from build123d import *

# Parameters (mm, degrees)
ESQUISSE1_W                  = 18.3
ESQUISSE1_H                  = 17.8
BOSS_EXTRU_1_DEPTH           = 34.4
ENL_V_MAT_EXTRU_1_DEPTH      = 37.69185877
ENL_V_MAT_EXTRU_1_DEPTH_BACK = 37.69185877
ENL_V_MAT_EXTRU_2_DEPTH      = 37.69185877
ENL_V_MAT_EXTRU_2_DEPTH_BACK = 37.69185877
ESQUISSE4_R                  = 4.25
BOSS_EXTRU_2_DEPTH           = 2.2
ESQUISSE5_R                  = 2.45
BOSS_EXTRU_3_DEPTH           = 2.1
BOSS_EXTRU_4_DEPTH           = 1.3
ESQUISSE7_R                  = 1.85
BOSS_EXTRU_5_DEPTH           = 10.3
ESQUISSE8_R                  = 6.5
ESQUISSE8_R_2                = 6.1
ENL_V_MAT_EXTRU_3_DEPTH      = 0.1


with BuildPart() as part:
    # Esquisse1 → Boss.-Extru.1 (new body)
    with BuildSketch(Plane(origin=(0, 0, 0), x_dir=(1, 0, 0), z_dir=(0, 1, 0))):
        Rectangle(ESQUISSE1_W, ESQUISSE1_H)
    extrude(amount=-BOSS_EXTRU_1_DEPTH)

    # Esquisse2 → Enlèv. mat.-Extru.1 (cut, two sides: drawn at the far end of the back side and taken through both)
    with BuildSketch(Plane(origin=(0, 0, 0), x_dir=(0, 0, -1), z_dir=(1, 0, 0)).offset(-ENL_V_MAT_EXTRU_1_DEPTH_BACK)):
        Polygon((8.9, -17.6), (4.4, -22.1), (4.4, -34.4), (8.9, -34.4), align=None)
    extrude(amount=ENL_V_MAT_EXTRU_1_DEPTH + ENL_V_MAT_EXTRU_1_DEPTH_BACK, mode=Mode.SUBTRACT)

    # Esquisse3 → Enlèv. mat.-Extru.2 (cut, two sides: drawn at the far end of the back side and taken through both)
    with BuildSketch(Plane.XY.offset(-ENL_V_MAT_EXTRU_2_DEPTH_BACK)):
        with BuildLine():
            Line((3.9, -30.7), (3.9, -25.7))
            ThreePointArc((3.9, -25.7), (5.4, -24.2), (6.9, -25.7))
            Line((6.9, -25.7), (6.9, -30.7))
            ThreePointArc((6.9, -30.7), (5.4, -32.2), (3.9, -30.7))
        make_face()
        with BuildLine():
            Line((-3.9, -30.7), (-3.9, -25.7))
            ThreePointArc((-3.9, -25.7), (-5.4, -24.2), (-6.9, -25.7))
            Line((-6.9, -25.7), (-6.9, -30.7))
            ThreePointArc((-6.9, -30.7), (-5.4, -32.2), (-3.9, -30.7))
        make_face()
    extrude(amount=ENL_V_MAT_EXTRU_2_DEPTH + ENL_V_MAT_EXTRU_2_DEPTH_BACK, mode=Mode.SUBTRACT)

    # Esquisse4 → Boss.-Extru.2 (add)
    with BuildSketch(Plane(origin=(0, 0, -4.4), x_dir=(-1, 0, 0), z_dir=(0, 0, -1))):
        with Locations((0, -19.85)):
            Circle(ESQUISSE4_R)
    extrude(amount=BOSS_EXTRU_2_DEPTH)

    # Esquisse5 → Boss.-Extru.3 (add)
    with BuildSketch(Plane(origin=(0, 0, -6.6), x_dir=(-1, 0, 0), z_dir=(0, 0, -1))):
        with Locations((0, -19.85)):
            Circle(ESQUISSE5_R)
    extrude(amount=BOSS_EXTRU_3_DEPTH)

    # Esquisse6 → Boss.-Extru.4 (add)
    with BuildSketch(Plane.XZ.offset(34.4)):
        with BuildLine():
            Line((3.75, 8.9), (3.75, 3.25))
            ThreePointArc((3.75, 3.25), (0, -0.5), (-3.75, 3.25))
            Line((-3.75, 3.25), (-3.75, 8.9))
            Line((-3.75, 8.9), (3.75, 8.9))
        make_face()
    extrude(amount=BOSS_EXTRU_4_DEPTH)

    # Esquisse7 → Boss.-Extru.5 (add)
    with BuildSketch(Plane.XZ.offset(35.7)):
        with Locations(Location((0, 3.25, 0), (0, 0, 90))):
            Circle(ESQUISSE7_R)
    extrude(amount=BOSS_EXTRU_5_DEPTH)

    # Esquisse8 → Enlèv. mat.-Extru.3 (cut)
    with BuildSketch(Plane(origin=(0, 0, 0), x_dir=(1, 0, 0), z_dir=(0, 1, 0))):
        with Locations(Location((0, 0, 0), (0, 0, 270))):
            Circle(ESQUISSE8_R)
        with Locations(Location((0, 0, 0), (0, 0, 270))):
            Circle(ESQUISSE8_R_2, mode=Mode.SUBTRACT)
    extrude(amount=-ENL_V_MAT_EXTRU_3_DEPTH, mode=Mode.SUBTRACT)


solid = part.part
Here's how the part is built. I have some questions about the finished solid (model axes, mm). A direction names the side the tool comes from. Give positions to 0.01 mm unless a question says otherwise; leave off trailing zeros. Order: outer loops, then holes, each group sorted by start corner. A loop starts at its lowest first (then second) coordinate and runs counter-clockwise, first axis right, second up. Notation, with made-up numbers: (-26.75, 23) -> (-14.75, 23) arc R22 cw to (-14.75, 30) -> close; hole circle Ø7 at (-8, 28.5). An arc over 180 degrees is marked (long way). One line per item, written item: value. Start each with the question number.
1. Imagine slicing it at A-A, the plane x = 0. List the corners of the cut face in (y, z) for me, plus the area to 3 significant figures.
2. Imagine slicing it at B-B, the plane z = 7.5. List the corners of the cut face in (x, y) for me.
3. I need wall thicknesses on probe 1 along X at (y, z) = (-0.05, 0); probe 2 along Z at (x, y) = (-6.75, -33); probe 3 along Y at (x, z) = (-7.75, 7.25). Which ranges of each line are inside material? Lowest first, please. Write a range as from..to.
4. Will these pins go through, and if not, where does the flat tip stop? pin 1 Ø10 at (x, y) = (0.5, -30.5) entering from -Z; pin 2 Ø6 at (x, z) = (-4.5, -6) entering from -Y; pin 3 Ø1.3 at (x, y) = (-1, -19) entering from -Z.
5. Imagine slicing it at C-C, the plane x = -5.4. List the corners of the cut face in (y, z) for me.
6. Imagine slicing it at D-D, the plane y = -42. List the corners of the cut face in (x, z) for me, plus the area to 3 significant figures.
7. For faces 1 (the face through (-3.9, -28, 2)), 2 (the face through (0, -20, -8.7)), 3 (the face through (-3.75, -35, 6)), 4 (the face through (0, -34.4, -1)), which set-ups out of +Z, -Z, +X, -X, +Y, -Y let a thin tool reach every point of the face, with its end or its side?
Values follow:
1. outline: (-46, 1.4) -> (-35.7, 1.4) -> (-35.7, -0.5) -> (-34.4, -0.5) -> (-34.4, -4.4) -> (-24.1, -4.4) -> (-24.1, -6.6) -> (-22.3, -6.6) -> (-22.3, -8.7) -> (-17.8, -8.7) -> (-17.6, -8.9) -> (0, -8.9) -> (0, -6.5) -> (-0.1, -6.5) -> (-0.1, -6.1) -> (0, -6.1) -> (0, 6.1) -> (-0.1, 6.1) -> (-0.1, 6.5) -> (0, 6.5) -> (0, 8.9) -> (-35.7, 8.9) -> (-35.7, 5.1) -> (-46, 5.1) -> close
1. area: 611 mm2
2. outline: (-9.15, -34.4) -> (-3.75, -34.4) -> (-3.75, -35.7) -> (3.75, -35.7) -> (3.75, -34.4) -> (9.15, -34.4) -> (9.15, 0) -> (-9.15, 0) -> close; hole (-6.9, -30.7) arc R1.5 ccw to (-3.9, -30.7) -> (-3.9, -25.7) arc R1.5 ccw to (-6.9, -25.7) -> close; hole (3.9, -30.7) arc R1.5 ccw to (6.9, -30.7) -> (6.9, -25.7) arc R1.5 ccw to (3.9, -25.7) -> close
3. probe 1: x = -9.15..-6.5, -6.1..6.1, 6.5..9.15
3. probe 2: z = -4.4..8.9
3. probe 3: y = -34.4..0
4. pin 1: stops at z = -4.4
4. pin 2: stops at y = -34.4
4. pin 3: stops at z = -8.7
5. outline: (-34.4, -4.4) -> (-32.2, -4.4) -> (-32.2, 8.9) -> (-34.4, 8.9) -> close; (-24.2, -4.4) -> (-22.1, -4.4) -> (-17.6, -8.9) -> (0, -8.9) -> (0, -3.62) -> (-0.1, -3.62) -> (-0.1, -2.84) -> (0, -2.84) -> (0, 2.84) -> (-0.1, 2.84) -> (-0.1, 3.62) -> (0, 3.62) -> (0, 8.9) -> (-24.2, 8.9) -> close
6. outline: circle Ø3.7 at (0, 3.25)
6. area: 10.8 mm2
7. face 1: +Z, -Z
7. face 2: -Z, +X, -X, -Y
7. face 3: +Z, -Z, -X, -Y
7. face 4: -Z, -Y
